Geometry check sheet. Reference: drawing and pictorial views, mm from the part's lowest x, y, z. A direction names the side the tool comes from. Give positions to 0.01 mm unless a question says otherwise; leave off trailing zeros. Write each loop counter-clockwise with the first axis right and the second up, starting at its lowest first coordinate (ties: lowest second). Pieces come first, ordered by that corner, then holes.
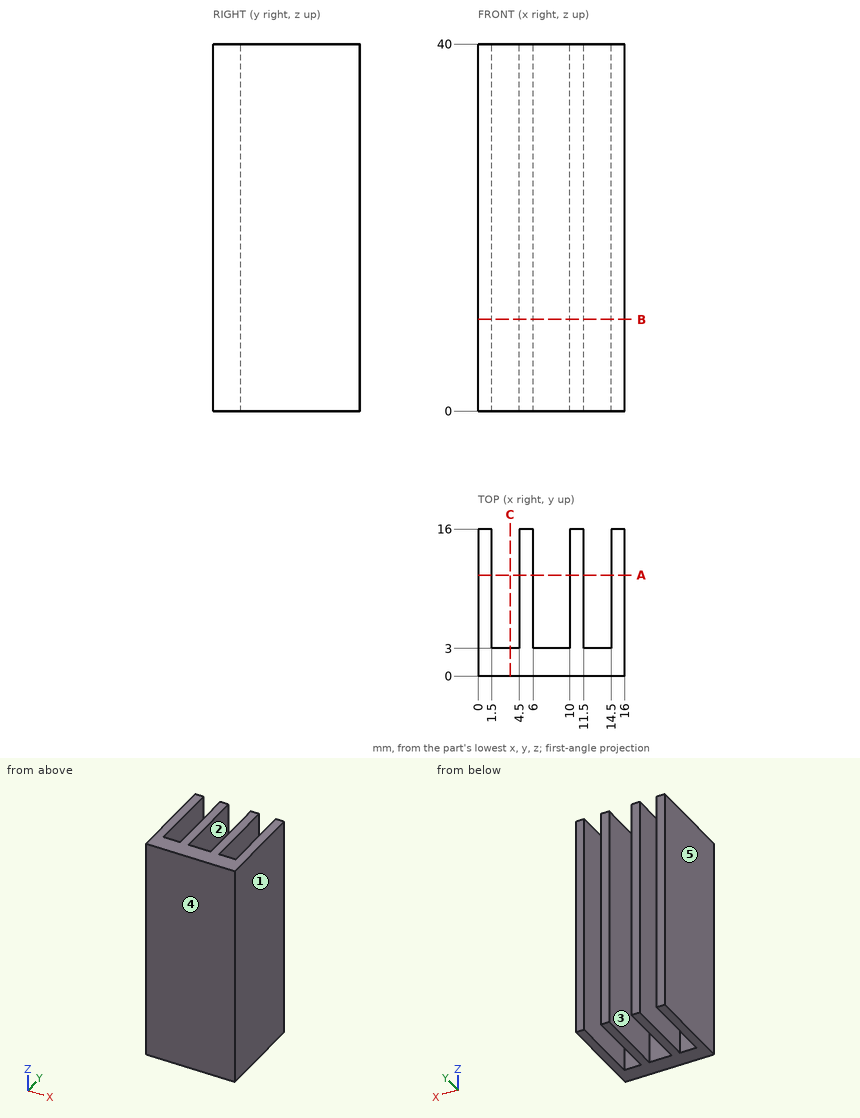
Item 1: Release check for a two-part mould opening along X. For the marked faces 3, 4 and 5 record: released by +X, released by -X, zero draft, split by the parting line, or undercut.
Answer key:
face 3: undercut
face 4: zero draft
face 5: released by -X
Item 2: Sectioned sample at A-A on y = 11. Record the cut outline in (x, z), then the cut area to 3 significant figures.
Answer key:
outline: (0, 0) - (1.5, 0) - (1.5, 40) - (0, 40) - close; (4.5, 0) - (6, 0) - (6, 40) - (4.5, 40) - close; (10, 0) - (11.5, 0) - (11.5, 40) - (10, 40) - close; (14.5, 0) - (16, 0) - (16, 40) - (14.5, 40) - close
area: 240 mm2
Item 3: Depth check by flat-ended pin: pin 1 (1.5 mm diameter, centred on x = 13, z = 23, fed in from +Y). Enter the tip coordinate at first touch or a pass-through.
Answer key:
pin 1: stops at y = 3
Item 4: Sectioned sample at C-C on x = 3.5. Record the cut outline in (y, z).
Answer key:
outline: (0, 0) - (3, 0) - (3, 40) - (0, 40) - close
Item 5: Sectioned sample at B-B on z = 10. Record the cut outline in (x, y).
Answer key:
outline: (0, 0) - (16, 0) - (16, 16) - (14.5, 16) - (14.5, 3) - (11.5, 3) - (11.5, 16) - (10, 16) - (10, 3) - (6, 3) - (6, 16) - (4.5, 16) - (4.5, 3) - (1.5, 3) - (1.5, 16) - (0, 16) - close
Item 6: Set-up check for the marked faces 1 and 2: record each of +Z, -Z, +X, -X, +Y, -Y from which the full face is reachable in a straight line by a thin tool's end or side.
Answer key:
face 1: +Z, -Z, +X, +Y, -Y
face 2: +Z, -Z, +Y
Item 7: Scan lines: line 1 along X through (y, z) = (4.75, 32.5); line 2 along Y through (x, z) = (3, 32.5). Record each from-to range of solid material in increasing order.
Answer key:
line 1: x = 0 to 1.5, 4.5 to 6, 10 to 11.5, 14.5 to 16
line 2: y = 0 to 3
